Check sheet for the modelled part. Datum: model origin and axes. Units: mm. Face numbers are marked on the shaded views. Round coordinates to 2 decimals unless told otherwise and drop trailing zeros. Order: outer loops, then holes, each group sorted by start corner. A loop starts at its lowest first (then second) coordinate and runs counter-clockwise, first axis right, second up.
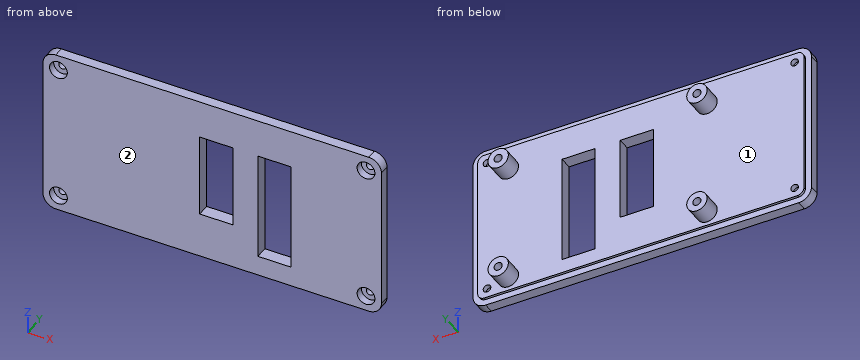
```python
from build123d import *

# Parameters (mm, degrees)
EXTRUDE_1_DEPTH     = 4
EXTRUDE_2_DEPTH     = 1
SKETCH_3_W          = 13
SKETCH_3_H          = 43
SKETCH_3_H_2        = 33
CUT_EXTRUDE_1_DEPTH = 6
SKETCH_4_R          = 4
SKETCH_4_R_2        = 1.6
EXTRUDE_4_DEPTH     = 7.3
SKETCH_5_R          = 1.5
CUT_EXTRUDE_2_DEPTH = 7.3
SKETCH_6_R          = 3.5
CUT_EXTRUDE_3_DEPTH = 3


with BuildPart() as part:
    # 스케치1 → 보스-돌출1 (new body)
    with BuildSketch(Plane(origin=(0, 0, 0), x_dir=(1, 0, 0), z_dir=(0, 1, 0))):
        with BuildLine():
            Line((61.498388188, 66.010476517), (-61.501611812, 65.989522963))
            ThreePointArc((-61.501611812, 65.989522963), (-65.036624731, 64.524771992), (-66.500805906, 60.989523028))
            Line((-66.500805906, 60.989523028), (-66.500805906, 4.989523158))
            ThreePointArc((-66.500805906, 4.989523158), (-65.03605487, 1.453704333), (-61.5, -0.010476777))
            Line((-61.5, -0.010476777), (61.5, 0.010476777))
            ThreePointArc((61.5, 0.010476777), (65.035012919, 1.475227749), (66.499194094, 5.010476712))
            Line((66.499194094, 5.010476712), (66.499194094, 61.010476582))
            ThreePointArc((66.499194094, 61.010476582), (65.034443058, 64.546295408), (61.498388188, 66.010476517))
        make_face()
    extrude(amount=EXTRUDE_1_DEPTH)

    # 스케치2 → 보스-돌출2 (add)
    with BuildSketch(Plane(origin=(0, 4, 0), x_dir=(1, 0, 0), z_dir=(0, 1, 0))):
        with BuildLine():
            Line((61.498751287, 63.610473876), (-61.501248713, 63.589525677))
            ThreePointArc((-61.501248713, 63.589525677), (-63.339440086, 62.827846783), (-64.100805906, 60.989525714))
            Line((-64.100805906, 60.989525714), (-64.100805906, 4.989525834))
            ThreePointArc((-64.100805906, 4.989525834), (-63.339126974, 3.150891653), (-61.500363098, 2.389525871))
            Line((-61.500363098, 2.389525871), (61.499636902, 2.410474071))
            ThreePointArc((61.499636902, 2.410474071), (63.337828275, 3.172152965), (64.099194094, 5.010474033))
            Line((64.099194094, 5.010474033), (64.099194094, 61.010473914))
            ThreePointArc((64.099194094, 61.010473914), (63.337515162, 62.849108095), (61.498751287, 63.610473876))
        make_face()
    extrude(amount=EXTRUDE_2_DEPTH)

    # 스케치3 → 컷-돌출1 (cut, through all)
    with BuildSketch(Plane(origin=(0, 5, 0), x_dir=(1, 0, 0), z_dir=(0, 1, 0))):
        with Locations((24.440725111, 36.53850122)):
            Rectangle(SKETCH_3_W, SKETCH_3_H)
        with Locations((1.580725111, 31.53850122)):
            Rectangle(SKETCH_3_W, SKETCH_3_H_2)
    extrude(amount=-CUT_EXTRUDE_1_DEPTH, mode=Mode.SUBTRACT)

    # 스케치4 → 보스-돌출4 (add)
    with BuildSketch(Plane(origin=(0, 5, 0), x_dir=(1, 0, 0), z_dir=(0, 1, 0))):
        with Locations((-26.042417718, 58.176282553)):
            Circle(SKETCH_4_R)
        with Locations((-26.042417718, 58.176282553)):
            Circle(SKETCH_4_R_2, mode=Mode.SUBTRACT)
        with Locations((52.062582282, 58.176282553)):
            Circle(SKETCH_4_R)
        with Locations((52.062582282, 58.176282553)):
            Circle(SKETCH_4_R_2, mode=Mode.SUBTRACT)
        with Locations((-26.042417718, 11.821282553)):
            Circle(SKETCH_4_R)
        with Locations((-26.042417718, 11.821282553)):
            Circle(SKETCH_4_R_2, mode=Mode.SUBTRACT)
        with Locations((52.062582282, 11.821282553)):
            Circle(SKETCH_4_R)
        with Locations((52.062582282, 11.821282553)):
            Circle(SKETCH_4_R_2, mode=Mode.SUBTRACT)
    extrude(amount=EXTRUDE_4_DEPTH)

    # 스케치5 → 컷-돌출2 (cut)
    with BuildSketch(Plane(origin=(0, 5, 0), x_dir=(1, 0, 0), z_dir=(0, 1, 0))):
        with Locations((60.440145734, 59.928842317)):
            Circle(SKETCH_5_R)
        with Locations((60.440145734, 6.092110978)):
            Circle(SKETCH_5_R)
        with Locations((-60.442726529, 59.928842317)):
            Circle(SKETCH_5_R)
        with Locations((-60.442726529, 6.092110978)):
            Circle(SKETCH_5_R)
    extrude(amount=-CUT_EXTRUDE_2_DEPTH, mode=Mode.SUBTRACT)

    # 스케치6 → 컷-돌출3 (cut)
    with BuildSketch(Plane.XZ):
        with Locations((60.450353981, -59.918545221)):
            Circle(SKETCH_6_R)
        with Locations((60.441182673, -6.081814663)):
            Circle(SKETCH_6_R)
        with Locations((-60.432516528, -59.939138113)):
            Circle(SKETCH_6_R)
        with Locations((-60.441687836, -6.102407556)):
            Circle(SKETCH_6_R)
    extrude(amount=-CUT_EXTRUDE_3_DEPTH, mode=Mode.SUBTRACT)


solid = part.part
```
Item 1: Go/stop test with flat-tipped pins: P1, Ø4, axis at x = 60.44, z = -59.93, coming from the -Y side; P2, Ø0.5, axis at x = -0.5, y = 4.5, coming from the +Z side; P3, Ø4, axis at x = 26.5, y = 3, coming from the +Z side. Record where each tip stops, or that it passes through.
Answer:
P1: stops at y = 3
P2: stops at z = -2.4
P3: stops at z = 0
Item 2: Sectioned sample at C-C (z = -51). Record the cut outline in (x, y).
Answer:
outline: (-66.5, 0) - (17.94, 0) - (17.94, 5) - (-64.1, 5) - (-64.1, 4) - (-66.5, 4) - close; (30.94, 0) - (66.5, 0) - (66.5, 4) - (64.1, 4) - (64.1, 5) - (30.94, 5) - close
Item 3: Sectioned sample at D-D (x = 23.5). Record the cut outline in (y, z).
Answer:
outline: (0, -66) - (4, -66) - (4, -63.6) - (5, -63.6) - (5, -58.04) - (0, -58.04) - close; (0, -15.04) - (5, -15.04) - (5, -2.4) - (4, -2.4) - (4, 0) - (0, 0) - close
Item 4: Release check for a two-part mould opening along X. For the marked faces 1 and 2 record: released by +X, released by -X, zero draft, split by the parting line, or undercut.
Answer:
face 1: undercut
face 2: zero draft
Item 5: Sectioned sample at B-B (y = 8.75). Record the cut outline in (x, z), and give its area (3 significant figures).
Answer:
outline: circle Ø8 at (-26.04, -58.18); circle Ø8 at (-26.04, -11.82); circle Ø8 at (52.06, -58.18); circle Ø8 at (52.06, -11.82); hole circle Ø3.2 at (-26.04, -58.18); hole circle Ø3.2 at (-26.04, -11.82); hole circle Ø3.2 at (52.06, -58.18); hole circle Ø3.2 at (52.06, -11.82)
area: 169 mm2
Item 6: Sectioned sample at A-A (z = -44). Record the cut outline in (x, y), and give its area (3 significant figures).
Answer:
outline: (-66.5, 0) - (-4.92, 0) - (-4.92, 5) - (-64.1, 5) - (-64.1, 4) - (-66.5, 4) - close; (8.08, 0) - (17.94, 0) - (17.94, 5) - (8.08, 5) - close; (30.94, 0) - (66.5, 0) - (66.5, 4) - (64.1, 4) - (64.1, 5) - (30.94, 5) - close
area: 530 mm2
Item 7: Scan lines: line 1 along X through (y, z) = (8.25, -12); line 2 along X through (y, z) = (0.75, -45); line 3 along Z through (x, y) = (51, 8.25) (1 decimal). Record each from-to range of solid material in increasing order.
Answer:
line 1: x = -30.04 to -27.63, -24.45 to -22.05, 48.07 to 50.47, 53.65 to 56.06
line 2: x = -66.5 to -4.92, 8.08 to 17.94, 30.94 to 66.5
line 3: z = -62 to -59.4, -57 to -54.3, -15.7 to -13, -10.6 to -8
